The drawing under review shows one solid part. Ordinate dimensions are in mm from its lowest x, y, z. Coordinates: 2 decimals unless noted, no trailing zeros. Write each loop counter-clockwise with the first axis right and the second up, starting at its lowest first coordinate (ties: lowest second). Pieces come first, ordered by that corner, then holes. Notation, with made-up numbers: (2, -35) - (51, -35) arc R15 cw to (51, -25) - close; hole circle Ø5 at (-34.5, -18.5). An arc over 180 degrees is marked (long way). Answer as CSV lines item,"result". Start each with the question number.
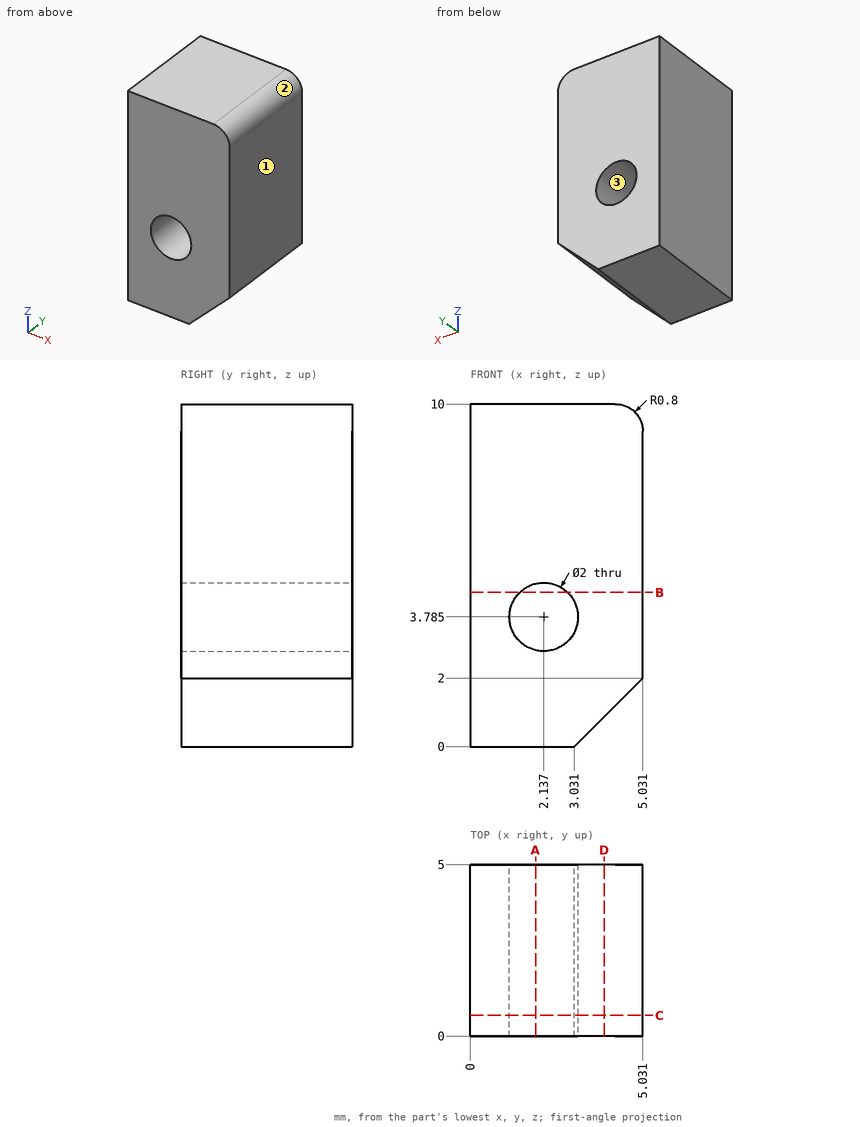
(1) Wall thickness on line 1 (Z direction, x = 2.1, y = 1.75) (1 decimal); line 2 (X direction, y = 0.4, z = 3.75); line 3 (Z direction, x = 2.5, y = 1.9) (1 decimal): over which ranges is each line inside the solid? List them lowest first.
(2) Add section D-D on x = 3.9. Give the boundary of the cut face in (y, z).
(3) The part is to be moulded in two halves that separate along Z. For the marked faces 1, 2 and 3, say which applies: released by +Z, released by -Z, zero draft, split by the parting line, or undercut.
(4) Add section A-A on x = 1.9. Give the boundary of the cut face in (y, z) (1 decimal).
(5) For pin 1 (1 mm diameter, centred on x = 4.5, y = 2.5, fed in from -Z); pin 2 (1.6 mm diameter, centred on x = 2.14, z = 3.79, fed in from -Y), all flat-tipped, find the tip position at first contact; note any pin that passes through.
(6) Add section C-C on y = 0.6. Give the boundary of the cut face in (x, z) (1 decimal).
(7) Add section B-B on z = 4.5. Give the boundary of the cut face in (x, y).
Reported:
1,line 1,"0 to 2.8, 4.8 to 10"
1,line 2,"0 to 1.14, 3.14 to 5.03"
1,line 3,"0 to 2.9, 4.7 to 10"
2,outline,"(0, 0.87) - (5, 0.87) - (5, 10) - (0, 10) - close"
3,face 1,"zero draft"
3,face 2,"released by +Z"
3,face 3,"undercut"
4,outline,"(0, 0) - (5, 0) - (5, 2.8) - (0, 2.8) - close; (0, 4.8) - (5, 4.8) - (5, 10) - (0, 10) - close"
5,pin 1,"z = 0.97"
5,pin 2,"through"
6,outline,"(0, 0) - (3, 0) - (5, 2) - (5, 9.2) arc R0.8 ccw to (4.2, 10) - (0, 10) - close; hole circle Ø2 at (2.1, 3.8)"
7,outline,"(0, 0) - (1.44, 0) - (1.44, 5) - (0, 5) - close; (2.84, 0) - (5.03, 0) - (5.03, 5) - (2.84, 5) - close"
